The listing builds one solid part. Answer for the finished solid, in the listing's coordinates (mm). Face numbers are marked on the shaded views. A direction names the side the tool comes from. Give positions to 0.01 mm unless a question says otherwise; leave off trailing zeros. Order: outer loops, then holes, each group sorted by start corner. A loop starts at its lowest first (then second) coordinate and runs counter-clockwise, first axis right, second up.
```python
from build123d import *

# Parameters (mm, degrees)
SKETCH5_W           = 190
SKETCH5_H           = 36
BOSS_EXTRUDE1_DEPTH = 8
SKETCH6_R           = 13
SKETCH6_R_2         = 12.99768992
CUT_EXTRUDE1_DEPTH  = 6
FILLET1_R           = 10
CUT_EXTRUDE2_DEPTH  = 8


with BuildPart() as part:
    # Sketch5 → Boss-Extrude1 (new body)
    with BuildSketch(Plane(origin=(0, 0, 0), x_dir=(1, 0, 0), z_dir=(0, 1, 0))):
        with Locations((95, 18)):
            Rectangle(SKETCH5_W, SKETCH5_H)
    extrude(amount=BOSS_EXTRUDE1_DEPTH)

    # Sketch6 → Cut-Extrude1 (cut)
    with BuildSketch(Plane(origin=(0, 8, 0), x_dir=(1, 0, 0), z_dir=(0, 1, 0))):
        with Locations(Location((23, 18, 0), (0, 0, 270))):
            Circle(SKETCH6_R)
        with Locations(Location((59, 18, 0), (0, 0, 270))):
            Circle(SKETCH6_R)
        with Locations(Location((95.004620161, 18, 0), (0, 0, 270))):
            Circle(SKETCH6_R)
        with Locations(Location((131.004620161, 18, 0), (0, 0, 270))):
            Circle(SKETCH6_R)
        with Locations(Location((167.00231008, 18, 0), (0, 0, 270))):
            Circle(SKETCH6_R_2)
    extrude(amount=-CUT_EXTRUDE1_DEPTH, mode=Mode.SUBTRACT)

    # Fillet1
    fillet1_edges = [part.edges().sort_by_distance(p)[0] for p in [
        (0, 4, -36),
        (190, 4, -36),
        (190, 4, 0),
        (0, 4, 0),
    ]]
    fillet(fillet1_edges, radius=FILLET1_R)

    # Sketch9 → Cut-Extrude2 (cut)
    with BuildSketch(Plane(origin=(0, 8, 0), x_dir=(1, 0, 0), z_dir=(0, 1, 0))):
        with BuildLine():
            Line((3.652564445, 7.899803831), (7.852564445, 7.899803831))
            Line((7.852564445, 7.899803831), (7.852564445, 3.699803831))
            ThreePointArc((7.852564445, 3.699803831), (3.324368465, 3.371607851), (3.652564445, 7.899803831))
        make_face()
        with BuildLine():
            Line((7.852564445, 28.100196169), (7.852564445, 32.300196169))
            ThreePointArc((7.852564445, 32.300196169), (3.324368465, 32.628392149), (3.652564445, 28.100196169))
            Line((3.652564445, 28.100196169), (7.852564445, 28.100196169))
        make_face()
        with BuildLine():
            Line((182.147435555, 7.899803831), (182.147435555, 3.699803831))
            ThreePointArc((182.147435555, 3.699803831), (186.675631535, 3.371607851), (186.347435555, 7.899803831))
            Line((186.347435555, 7.899803831), (182.147435555, 7.899803831))
        make_face()
        with BuildLine():
            Line((182.147435555, 28.100196169), (182.147435555, 32.300196169))
            ThreePointArc((182.147435555, 32.300196169), (186.675631535, 32.628392149), (186.347435555, 28.100196169))
            Line((186.347435555, 28.100196169), (182.147435555, 28.100196169))
        make_face()
    extrude(amount=-CUT_EXTRUDE2_DEPTH, mode=Mode.SUBTRACT)


solid = part.part
```
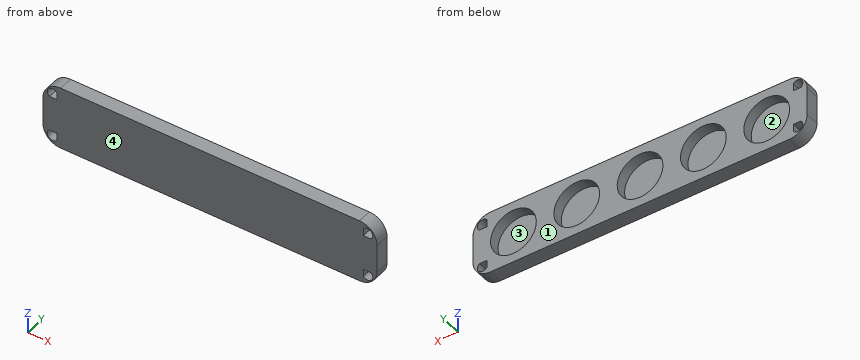
1) Find section B-B (z = -18). Write down the section's boundary in (x, y), then the cut area to 3 significant figures.
Geometry says:
outline: (0, 0) - (190, 0) - (190, 8) - (180, 8) - (180, 2) - (154, 2) - (154, 8) - (144, 8) - (144, 2) - (118, 2) - (118, 8) - (108, 8) - (108, 2) - (82, 2) - (82, 8) - (72, 8) - (72, 2) - (46, 2) - (46, 8) - (36, 8) - (36, 2) - (10, 2) - (10, 8) - (0, 8) - close
area: 740 mm2
2) For a pull along Z with two mould halves and no side action, classify the marked faces 3 and 4 as +Z half, -Z half, draft (parallel to the pull), parting line (faces both ways), or undercut.
Geometry says:
face 3: undercut
face 4: draft
3) Given P1, Ø21, axis at x = 23, z = -18, coming from the +Y side; P2, Ø1.3, axis at y = 3.5, z = -5, coming from the -X side; P3, Ø1.3, axis at x = 5.5, y = 2.5, coming from the -Z side, each flat-ended and moving along its own axis, determine where each tip first touches the part or whether it passes through.
Geometry says:
P1: stops at y = 2
P2: stops at x = 1
P3: stops at z = -35.23
4) Straight lines are drawn through the part: probe 1 along X at (y, z) = (5.5, -18); probe 2 along X at (y, z) = (7.5, -3); probe 3 along Y at (x, z) = (106, -13). For each, find the intervals that lie inside material, in ascending order.
Geometry says:
probe 1: x = 0 to 10, 36 to 46, 72 to 82, 108 to 118, 144 to 154, 180 to 190
probe 2: x = 2.86 to 3.78, 7.12 to 182.88, 186.22 to 187.14
probe 3: y = 0 to 2
5) Find section C-C (x = 59). Write down the section's boundary in (y, z).
Geometry says:
outline: (0, -36) - (8, -36) - (8, -31) - (2, -31) - (2, -5) - (8, -5) - (8, 0) - (0, 0) - close
6) Find section D-D (x = 175). Write down the section's boundary in (y, z), then the cut area to 3 significant figures.
Geometry says:
outline: (0, -36) - (8, -36) - (8, -28.25) - (2, -28.25) - (2, -7.75) - (8, -7.75) - (8, 0) - (0, 0) - close
area: 165 mm2
7) Find section A-A (y = 5.5). Count the separate pieces of the cut face and the enclosed holes in it, then the cut area to 3 significant figures.
Geometry says:
separate pieces: 1
enclosed holes: 9
area: 4,000 mm2
8) A tool of negligible diameter and unlimited length cuts with its end or side. For the marked faces 1 and 2, from which of +Z, -Z, +X, -X, +Y, -Y can it reach the whole face along a straight path? Write none if from no direction.
Geometry says:
face 1: +Z, -Z, +X, -X, +Y
face 2: +Y
